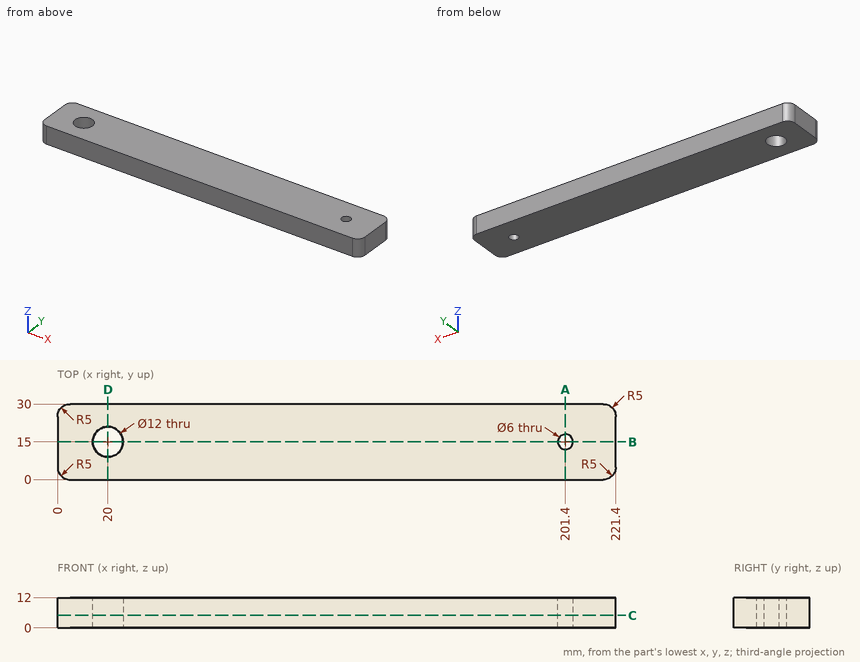
Here's the drawing with two shaded views (mm, measured from the low corner). I have some questions. Round coordinates to 2 decimals unless told otherwise and drop trailing zeros. Loops run counter-clockwise (first coordinate to the right, second up) from the corner with the lowest first, then second, coordinate; pieces in that order, holes last. Notation, with made-up numbers: M -1,34 L 48,34 A7 cw 48,39 Z; hole C 61.25,-33 d6. An arc over 180 degrees is marked long. Answer as CSV lines item,"result".
1) Imagine slicing it at A-A on x = 201.4. List the corners of the cut face in (y, z) for me.
From the geometry:
outline,"M 0,0 L 12,0 L 12,12 L 0,12 Z; M 18,0 L 30,0 L 30,12 L 18,12 Z"
2) Imagine slicing it at D-D on x = 20. List the corners of the cut face in (y, z) for me.
From the geometry:
outline,"M 0,0 L 9,0 L 9,12 L 0,12 Z; M 21,0 L 30,0 L 30,12 L 21,12 Z"
3) Imagine slicing it at B-B on y = 15. List the corners of the cut face in (x, z) for me.
From the geometry:
outline,"M 0,0 L 14,0 L 14,12 L 0,12 Z; M 26,0 L 198.4,0 L 198.4,12 L 26,12 Z; M 204.4,0 L 221.4,0 L 221.4,12 L 204.4,12 Z"
4) If I drill on probe 1 along Y at (x, z) = (201.4, 8.25); probe 2 along Y at (x, z) = (20, 7); probe 3 along X at (y, z) = (15.25, 10.5), over which ranges is the centre line in solid material (lowest first)?
From the geometry:
probe 1,"0 to 12, 18 to 30"
probe 2,"0 to 9, 21 to 30"
probe 3,"0 to 14.01, 25.99 to 198.41, 204.39 to 221.4"
5) Imagine slicing it at C-C on z = 5. List the corners of the cut face in (x, y) for me, and give its area (3 significant figures).
From the geometry:
outline,"M 0,5 A5 ccw 5,0 L 216.4,0 A5 ccw 221.4,5 L 221.4,25 A5 ccw 216.4,30 L 5,30 A5 ccw 0,25 Z; hole C 20,15 d12; hole C 201.4,15 d6"
area,"6,480 mm^2"
